from build123d import *

# Parameters (mm, degrees)
F1_DEPTH = 7.5
F3_D     = 20
F4_D     = 10


with BuildPart() as f1:
    # F0 (on Front) → F1 (new body, symmetric)
    with BuildSketch(Plane.XZ):
        with BuildLine():
            Line((9.9498743711, -101), (19.8997487421, -2))
            ThreePointArc((19.8997487421, -2), (0, 20), (-19.8997487421, -2))
            Line((-19.8997487421, -2), (-9.9498743711, -101))
            ThreePointArc((-9.9498743711, -101), (0, -110), (9.9498743711, -101))
        make_face()
    extrude(amount=F1_DEPTH, both=True)

    # F3 (through all)
    with Locations(Plane.XZ.offset(7.5)):
        with Locations((0, 0)):
            Hole(F3_D / 2)

    # F4 (through all)
    with Locations(Plane.XZ.offset(7.5)):
        with Locations((0, -100)):
            Hole(F4_D / 2)


solid = f1.part
Part model, mm, in its own coordinate system. Coordinates: 2 decimals unless noted, no trailing zeros. Order: outer loops, then holes, each group sorted by start corner. A loop starts at its lowest first (then second) coordinate and runs counter-clockwise, first axis right, second up.
(1) Probe L1, parallel to Z at x = 0.5, y = -7; L2, parallel to Z at x = 4, y = -4.5; L3, parallel to X at y = 3.25, z = 8. List the from-to ranges inside material, lowest first.
Check sheet entries:
L1: z = -109.99 to -104.97, -95.03 to -9.99, 9.99 to 19.99
L2: z = -109.17 to -103, -97 to -9.17, 9.17 to 19.6
L3: x = -18.33 to -6, 6 to 18.33
(2) Slice it at B-B, the plane z = 0. Write the cut outline in (x, y).
Check sheet entries:
outline: (-20, -7.5) - (-10, -7.5) - (-10, 7.5) - (-20, 7.5) - close; (10, -7.5) - (20, -7.5) - (20, 7.5) - (10, 7.5) - close
(3) Pull direction X, two halves, no side cores. Call faces 1 (the face through (0, 0, -110)), 2 (the face through (-14.994, -0.105, -50.807)), 3 (the face through (1.08, 0.1, -104.88)), 4 (the face through (0, 7.5, -44)): pulls with the +X half, pulls with the -X half, needs draft (parallel to the pull), parting line crosses it, or undercut.
Check sheet entries:
face 1: parting line crosses it
face 2: pulls with the -X half
face 3: undercut
face 4: needs draft
(4) Slice it at A-A, the plane x = 0. Write the cut outline in (y, z).
Check sheet entries:
outline: (-7.5, -110) - (7.5, -110) - (7.5, -105) - (-7.5, -105) - close; (-7.5, -95) - (7.5, -95) - (7.5, -10) - (-7.5, -10) - close; (-7.5, 10) - (7.5, 10) - (7.5, 20) - (-7.5, 20) - close
(5) Slice it at C-C, the plane y = 1.5. Write the cut outline in (x, z), and give its area (3 significant figures).
Check sheet entries:
outline: (-19.9, -2) - (-9.95, -101) arc R10 ccw to (9.95, -101) - (19.9, -2) arc R20 ccw (long way) to start; hole circle Ø20 at (0, 0); hole circle Ø10 at (0, -100)
area: 3,410 mm2
(6) Slice it at D-D, the plane x = -7. Write the cut outline in (y, z) (3 decimals).
Check sheet entries:
outline: (-7.5, -107.141) - (7.5, -107.141) - (7.5, -7.141) - (-7.5, -7.141) - close; (-7.5, 7.141) - (7.5, 7.141) - (7.5, 18.735) - (-7.5, 18.735) - close
(7) Pin check, flat tips, straight feed: pin 1 Ø8 at (x, y) = (9.5, -4.5) entering from +Z; pin 2 Ø1.5 at (x, y) = (8, 3) entering from -Z; pin 3 Ø1.5 at (y, z) = (3, -74.5) entering from +X; pin 4 Ø16 at (x, z) = (0, -100) entering from -Y. Stop position of each tip, or through.
Check sheet entries:
pin 1: stops at z = 19.23
pin 2: stops at z = -106.89
pin 3: stops at x = 12.69
pin 4: stops at y = -7.5
